from build123d import *

# Parameters (mm, degrees)
F1_DEPTH = 152.4
F2_R     = 5
F3_W     = 142.4
F3_H     = 33.168938
F3_W_2   = 134.4
F3_H_2   = 25.168938
F4_DEPTH = 4
F5_R     = 1


with BuildPart() as f1:
    # F0 (on Right) → F1 (new body)
    with BuildSketch(Plane.YZ):
        Polygon((-22.256978, -83.947913), (0, -83.947913), (22.256978, -83.947913), (9.401655, 17.652087), (0, 17.652087), (-9.401655, 17.652087), align=None)
    extrude(amount=F1_DEPTH)

    # F2
    f2_edges = [f1.edges().sort_by_distance(p)[0] for p in [
        (76.2, 22.256978, -83.947913),
        (76.2, 9.401655, 17.652087),
        (0, 15.829316, -33.147913),
        (152.4, 15.829316, -33.147913),
        (76.2, -9.401655, 17.652087),
        (76.2, -22.256978, -83.947913),
        (0, -15.829316, -33.147913),
        (152.4, -15.829316, -33.147913),
        (152.4, 0, 17.652087),
        (0, 0, 17.652087),
        (152.4, 0, -83.947913),
        (0, 0, -83.947913),
    ]]
    fillet(f2_edges, radius=F2_R)

    # F3 (on face) → F4 (join)
    with BuildSketch(Plane(origin=(0, 0, -83.947913), x_dir=(1, 0, 0), z_dir=(0, 0, -1))):
        with Locations((76.2, 0)):
            Rectangle(F3_W, F3_H)
        with Locations((76.2, 0)):
            Rectangle(F3_W_2, F3_H_2, mode=Mode.SUBTRACT)
    extrude(amount=F4_DEPTH)

    # F5
    f5_edges = [f1.edges().sort_by_distance(p)[0] for p in [
        (147.4, 0, -87.947913),
        (76.2, -16.584469, -87.947913),
        (5, 0, -87.947913),
        (76.2, 16.584469, -87.947913),
        (9, 0, -87.947913),
        (76.2, -12.584469, -87.947913),
        (143.4, 0, -87.947913),
        (76.2, 12.584469, -87.947913),
    ]]
    fillet(f5_edges, radius=F5_R)


solid = f1.part
Part model, mm, in its own coordinate system. A direction names the side the tool comes from. Round coordinates to 2 decimals unless told otherwise and drop trailing zeros. Write each loop counter-clockwise with the first axis right and the second up, starting at its lowest first coordinate (ties: lowest second). Pieces come first, ordered by that corner, then holes. Notation, with made-up numbers: (27.5, -26) - (44.5, -26) arc R25 cw to (44.5, -7) - close; hole circle Ø4 at (53.25, 4.5). An arc over 180 degrees is marked (long way). Use CSV: the item, a comma, the result in double quotes.
Item 1: Flat gauge pins, fed straight in: P1, Ø1.5, axis at y = 7, z = -86, coming from the +X side; P2, Ø10, axis at x = 94.5, z = 2.5, coming from the +Y side; P3, Ø1.5, axis at x = 71, z = -85, coming from the +Y side. Where does each tip first touch, or does it go through?
Results list:
P1,"stops at x = 147.4"
P2,"stops at y = 11.95"
P3,"stops at y = 16.58"
Item 2: Pull direction X, two halves, no side cores. Call faces 4 (the flat face through (75, -12.584, -85)), 5 (the cylindrical face through (1.5, 0.23, -82.52)), 6 (the cylindrical face through (150.9, 14.25, -32.06)), 7 (the flat face through (75, 0, 17.652)): pulls with the +X half, pulls with the -X half, needs draft (parallel to the pull), parting line crosses it, or undercut.
Results list:
face 4,"undercut"
face 5,"pulls with the -X half"
face 6,"pulls with the +X half"
face 7,"needs draft"
Item 3: Slice it at A-A, the plane y = 3. Write the cut outline in (x, z), then the cut area to 3 significant figures.
Results list:
outline,"(0, -78.95) arc R5 ccw to (5, -83.95) - (5, -86.95) arc R1 ccw to (6, -87.95) - (8, -87.95) arc R1 ccw to (9, -86.95) - (9, -83.95) - (143.4, -83.95) - (143.4, -86.95) arc R1 ccw to (144.4, -87.95) - (146.4, -87.95) arc R1 ccw to (147.4, -86.95) - (147.4, -83.95) arc R5 ccw to (152.4, -78.95) - (152.4, 12.65) arc R5 ccw to (147.4, 17.65) - (5, 17.65) arc R5 ccw to (0, 12.65) - close"
area,"15,500 mm²"
Item 4: Slice it at B-B, the plane x = 67.5. Write the cut outline in (y, z).
Results list:
outline,"(-21.54, -78.32) arc R5 ccw to (-16.58, -83.95) - (-16.58, -86.95) arc R1 ccw to (-15.58, -87.95) - (-13.58, -87.95) arc R1 ccw to (-12.58, -86.95) - (-12.58, -83.95) - (12.58, -83.95) - (12.58, -86.95) arc R1 ccw to (13.58, -87.95) - (15.58, -87.95) arc R1 ccw to (16.58, -86.95) - (16.58, -83.95) arc R5 ccw to (21.54, -78.32) - (9.95, 13.28) arc R5 ccw to (4.99, 17.65) - (-4.99, 17.65) arc R5 ccw to (-9.95, 13.28) - close"
Item 5: Wall check: L1, parallel to Z at x = 92.5, y = 1.5; L2, parallel to X at y = 14, z = -55.5; L3, parallel to Y at x = 114, z = -79.5. Give the ranges that are in metal, low to high.
Results list:
L1,"z = -83.95 to 17.65"
L2,"x = 0.01 to 152.39"
L3,"y = -21.55 to 21.55"
Item 6: Tool access for faces 1 (the flat face through (147.4, 0, -85)), 2 (the flat face through (75, 16.584, -85)), 3 (the flat face through (75, -16.584, -85)): list every direction of +Z, -Z, +X, -X, +Y, -Y with a clear straight run to the whole face (end or side of a thin tool).
Results list:
face 1,"-Z, +X, +Y, -Y"
face 2,"-Z, +X, -X, +Y"
face 3,"-Z, +X, -X, -Y"
